Input: part model. Units: mm. Frame: model coordinates. Face numbers are marked on the shaded views. A direction names the side the tool comes from. Give positions to 0.01 mm unless a question says otherwise; leave off trailing zeros. Loops run counter-clockwise (first coordinate to the right, second up) from the corner with the lowest first, then second, coordinate; pieces in that order, holes last. Notation, with made-up numbers: M 88,78.5 L 134,78.5 A21 cw 134,99.5 Z; hole C 54.25,77.25 d1. An arc over 180 degrees is marked long. One line per item, written item: value. Start each with the question number.
(1) Ray query, line 1 along Y through (x, z) = (-70, -13); line 2 along Z through (x, y) = (-79.5, -24); line 3 along X through (y, z) = (-35, 12.5). Return the intervals inside material, ascending. Write a range as from..to.
(2) Access query for the marked faces 5, 6 and 7. Directions: +Z, -Z, +X, -X, +Y, -Y. A direction counts if a zero-diameter tool reaches every point of the face in a straight line with its end or side. Return the directions, or none.
(3) Pull-direction query (Y, two-part tool) for the marked faces 1, 2, 3 and 4; classes: released by +Y, released by -Y, zero draft, split by the parting line, or undercut.
(4) Pin query (flat end, axial travel): P1, Ø1, axis at y = -21, z = -1.5, coming from the +X side; P2, Ø13.5, axis at x = -71.06, y = -15, coming from the +Z side; P3, Ø10, axis at x = -63, y = -8.5, coming from the +Z side; P4, Ø10, axis at x = -50.5, y = -16.5, coming from the +Z side. Return the tip coordinate at first contact, or that it passes through.
(5) Section B-B on x = -34.5. Output: boundary loops of the cut face in (y, z), plus the area to 3 significant figures.
(6) Section D-D on y = -32.5. Output: boundary loops of the cut face in (x, z), plus the area to 3 significant figures.
(7) Section A-A on x = -17.5. Output: boundary loops of the cut face in (y, z).
(8) Section C-C on y = -15. Output: boundary loops of the cut face in (x, z), plus the area to 3 significant figures.
```python
from build123d import *

# Parameters (mm, degrees)
SKETCH1_W           = 80
SKETCH1_H           = 10
BOSS_EXTRUDE1_DEPTH = 40
SKETCH3_W           = 80
SKETCH3_H           = 10
BOSS_EXTRUDE2_DEPTH = 40
BOSS_EXTRUDE6_DEPTH = 30
SKETCH8_R           = 7.5
CUT_EXTRUDE1_DEPTH  = 10
SKETCH9_R           = 7.5
CUT_EXTRUDE2_DEPTH  = 30
FILLET1_R           = 10
SKETCH10_R          = 7.5
CUT_EXTRUDE3_DEPTH  = 12


with BuildPart() as part:
    # Sketch1 → Boss-Extrude1 (new body)
    with BuildSketch(Plane(origin=(0, 0, 0), x_dir=(1, 0, 0), z_dir=(0, 1, 0))):
        with Locations((-45.97826087, 19.239130435)):
            Rectangle(SKETCH1_W, SKETCH1_H)
    extrude(amount=-BOSS_EXTRUDE1_DEPTH)

    # Sketch3 → Boss-Extrude2 (add)
    with BuildSketch(Plane.XY.offset(-14.239130435)):
        with Locations((-45.97826087, -35)):
            Rectangle(SKETCH3_W, SKETCH3_H)
    extrude(amount=BOSS_EXTRUDE2_DEPTH)

    # Sketch7 → Boss-Extrude6 (add)
    with BuildSketch(Plane(origin=(0, -30, 0), x_dir=(1, 0, 0), z_dir=(0, 1, 0))):
        Polygon((-35.97826087, 14.239130435), (-45.97826087, 14.239130435), (-66.731833313, -21.707111476), (-58.312851229, -25.760869565), align=None)
    extrude(amount=BOSS_EXTRUDE6_DEPTH)

    # Sketch8 → Cut-Extrude1 (cut)
    with BuildSketch(Plane(origin=(0, -30, 0), x_dir=(1, 0, 0), z_dir=(0, 1, 0))):
        with Locations(Location((-18.3763958, -10.760869565, 0), (0, 0, 270))):
            Circle(SKETCH8_R)
        with Locations(Location((-75.358914669, -10.760869565, 0), (0, 0, 270))):
            Circle(SKETCH8_R)
    extrude(amount=-CUT_EXTRUDE1_DEPTH, mode=Mode.SUBTRACT)

    # Sketch9 → Cut-Extrude2 (cut)
    with BuildSketch(Plane.XY.offset(-14.239130435)):
        with Locations((-20.97826087, -15)):
            Circle(SKETCH9_R)
        with Locations((-71.057215434, -15)):
            Circle(SKETCH9_R)
    extrude(amount=-CUT_EXTRUDE2_DEPTH, mode=Mode.SUBTRACT)

    # Fillet1
    fillet1_edges = [part.edges().sort_by_distance(p)[0] for p in [
        (-5.97826087, -35, 25.760869565),
        (-85.97826087, -35, 25.760869565),
        (-62.522342271, 0, 23.733990521),
        (-85.97826087, 0, -19.239130435),
        (-5.97826087, 0, -19.239130435),
    ]]
    fillet(fillet1_edges, radius=FILLET1_R)

    # Sketch10 → Cut-Extrude3 (cut)
    with BuildSketch(Plane(origin=(-33.488225208, 0, -18.698644797), x_dir=(0.48751608982422123, 0, -0.873114002958664), z_dir=(0.873114002958664, 0, 0.48751608982422123))):
        with Locations((-27.107596885, -15)):
            Circle(SKETCH10_R)
    extrude(amount=-CUT_EXTRUDE3_DEPTH, mode=Mode.SUBTRACT)


solid = part.part
```
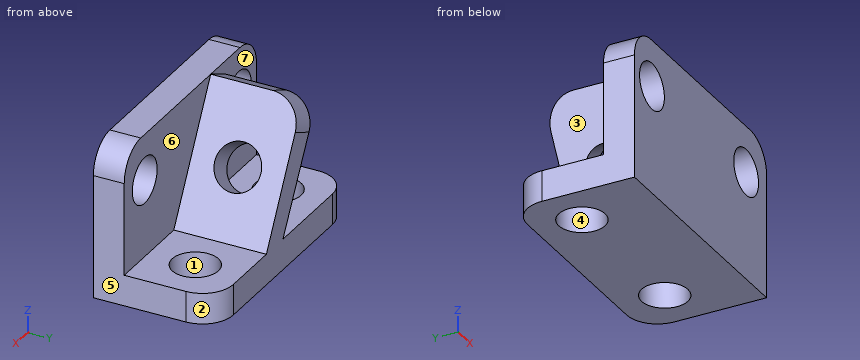
Output values:
1. line 1: y = -40..-30
1. line 2: z = -24.24..-14.24
1. line 3: x = -85.98..-82.65, -68.06..-25.67, -11.08..-5.98
2. face 5: +Z, -Z, +X, +Y, -Y
2. face 6: +Z, +X, +Y
2. face 7: -X, +Y
3. face 1: undercut
3. face 2: released by +Y
3. face 3: zero draft
3. face 4: undercut
4. P1: stops at x = -42.81
4. P2: stops at z = 22.87
4. P3: stops at z = 25.76
4. P4: stops at z = 20.72
5. outline: M -40,-24.24 L 0,-24.24 L 0,-14.24 L -30,-14.24 L -30,25.76 L -40,25.76 Z
5. area: 800 mm²
6. outline: M -85.98,-24.24 L -5.98,-24.24 L -5.98,15.76 A10 ccw -15.98,25.76 L -75.98,25.76 A10 ccw -85.98,15.76 Z; hole C -75.36,10.76 d15; hole C -18.38,10.76 d15
6. area: 3,600 mm²
7. outline: M -40,-24.24 L -21.64,-24.24 L -21.64,-14.24 L -30,-14.24 L -30,3.31 L -40,3.31 Z; M -40,18.21 L -30,18.21 L -30,25.76 L -40,25.76 Z; M -8.36,-24.24 L 0,-24.24 L 0,-14.24 L -8.36,-14.24 Z
8. outline: M -85.98,-24.24 L -78.56,-24.24 L -78.56,-14.24 L -85.98,-14.24 Z; M -66.73,21.71 L -58.29,7.09 L -50.36,11.52 L -58.31,25.76 Z; M -63.56,-24.24 L -28.48,-24.24 L -28.48,-14.24 L -35.98,-14.24 L -43.05,-1.58 L -50.79,-5.9 L -45.98,-14.24 L -63.56,-14.24 Z; M -13.48,-24.24 L -5.98,-24.24 L -5.98,-14.24 L -13.48,-14.24 Z
8. area: 759 mm²
